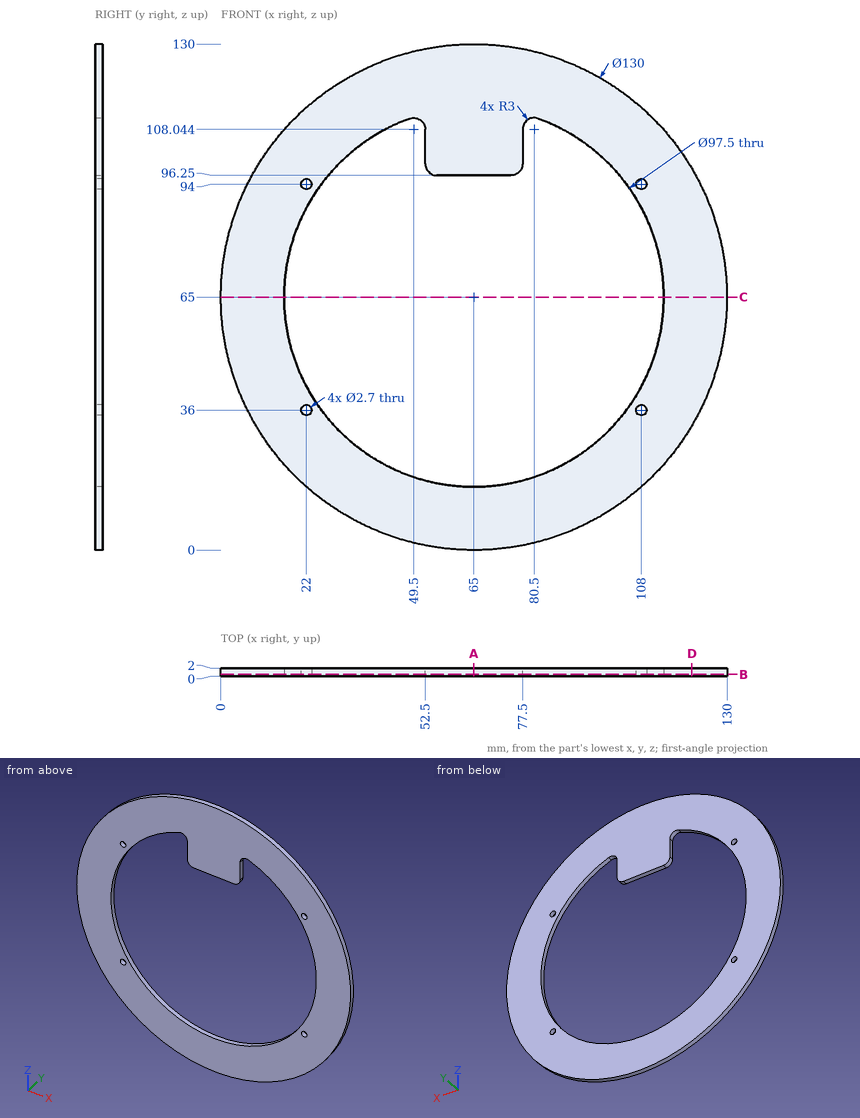
For this review, use the dimensioned drawing (mm, ordinates from the lowest corner) and the shaded views. Give positions to 0.01 mm unless a question says otherwise; leave off trailing zeros. Order: outer loops, then holes, each group sorted by start corner. A loop starts at its lowest first (then second) coordinate and runs counter-clockwise, first axis right, second up. Notation, with made-up numbers: (56, 31) - (98, 31) arc R22 ccw to (98, 66) - close; hole circle Ø8 at (12.5, 26.25). An arc over 180 degrees is marked (long way). Use a Markdown table: item, result. Add a question column.
(1) Add section A-A on x = 65. Give the boundary of the cut face in (y, z).
(2) Add section B-B on y = 0.4. Give the boundary of the cut face in (x, z).
(3) Wall thickness on probe 1 along X at (y, z) = (0.3, 101.5) (1 decimal); probe 2 along X at (y, z) = (1.8, 94.5) (1 decimal); probe 3 along X at (y, z) = (1.85, 106) (1 decimal): over which ranges is each line inside the solid? List them lowest first. Write a range as [from, to].
(4) Add section D-D on x = 121. Give the boundary of the cut face in (y, z).
(5) Add section C-C on z = 65. Give the boundary of the cut face in (x, y).
(6) Clearance check with flat-ended pins moving along their axes: P1, Ø1.6, axis at x = 108, z = 36, coming from the -Y side; P2, Ø4.5, axis at x = 108, z = 94, coming from the -Y side; P3, Ø0.6, axis at y = 0.5, z = 102.5, coming from the -X side; P4, Ø0.6, axis at y = 1, z = 103.5, coming from the +X side. State where each tip first meets the part, or that it passes through.
Report:
| question | item | result |
|---|---|---|
| 1 | outline | (0, 0) - (2, 0) - (2, 16.25) - (0, 16.25) - close; (0, 96.25) - (2, 96.25) - (2, 130) - (0, 130) - close |
| 2 | outline | circle Ø130 at (65, 65); hole circle Ø2.7 at (22, 36); hole circle Ø2.7 at (22, 94); hole (48.48, 110.87) arc R48.75 ccw (long way) to (81.52, 110.87) arc R3 ccw to (77.5, 108.04) - (77.5, 99.25) arc R3 cw to (74.5, 96.25) - (55.5, 96.25) arc R3 cw to (52.5, 99.25) - (52.5, 108.04) arc R3 ccw to start; hole circle Ø2.7 at (108, 36); hole circle Ø2.7 at (108, 94) |
| 3 | probe 1 | x = [11.2, 32.7], [52.5, 77.5], [97.3, 118.8] |
| 3 | probe 2 | x = [7.1, 20.7], [23.3, 26.2], [103.8, 106.7], [109.3, 122.9] |
| 3 | probe 3 | x = [14.6, 38.6], [52.5, 77.5], [91.4, 115.4] |
| 4 | outline | (0, 32) - (2, 32) - (2, 98) - (0, 98) - close |
| 5 | outline | (0, 0) - (16.25, 0) - (16.25, 2) - (0, 2) - close; (113.75, 0) - (130, 0) - (130, 2) - (113.75, 2) - close |
| 6 | P1 | passes through |
| 6 | P2 | stops at y = 0 |
| 6 | P3 | stops at x = 11.7 |
| 6 | P4 | stops at x = 117.59 |
